Could you check a few things on this drawing? It's one solid part, dimensions in mm from its lowest x, y, z. Give positions to 0.01 mm unless a question says otherwise; leave off trailing zeros. Write each loop counter-clockwise with the first axis right and the second up, starting at its lowest first coordinate (ties: lowest second). Pieces come first, ordered by that corner, then holes. Notation, with made-up numbers: (68, -27) -> (79, -27) arc R31 ccw to (79, 7) -> close; hole circle Ø2 at (-31, -37.75). An arc over 180 degrees is marked (long way). Use CSV: the item, a comma, the result in double quotes. Start each with the question number.
(1) For pin 1 Ø1 at (x, y) = (23.5, 11.5) entering from -Z; pin 2 Ø8 at (x, z) = (10.5, 18) entering from +Y; pin 3 Ø6 at (y, z) = (9, 27) entering from -X; pin 4 Ø6 at (x, z) = (4.5, 11.5) entering from -Y, each with a flat end and sliding along its axis, tell me the tip position at first contact or that it passes through.
(2) Suppose I cut it at D-D on y = 3.5. List the corners of the cut face in (x, z) for me.
(3) Suppose I cut it at C-C on y = 26. List the corners of the cut face in (x, z) for me, plus the area to 3 significant figures.
(4) Suppose I cut it at A-A on x = 17. List the corners of the cut face in (y, z) for me, plus the area to 3 significant figures.
(5) I need wall thicknesses on L1, parallel to X at y = 14.5, z = 17; L2, parallel to Y at x = 12.5, z = 4.5; L3, parallel to Z at x = 10, y = 28. Which ranges of each line are inside material? Lowest first, please. Write a range as [from, to].
(6) If we mould it in two halves opening along Z, with no side actions, what happens to the marked faces 1, 2 and 3? For each: pulls with the +Z half, pulls with the -Z half, needs draft (parallel to the pull), parting line crosses it, or undercut.
(7) Suppose I cut it at B-B on z = 17. List the corners of the cut face in (x, y) for me, plus the area to 3 significant figures.
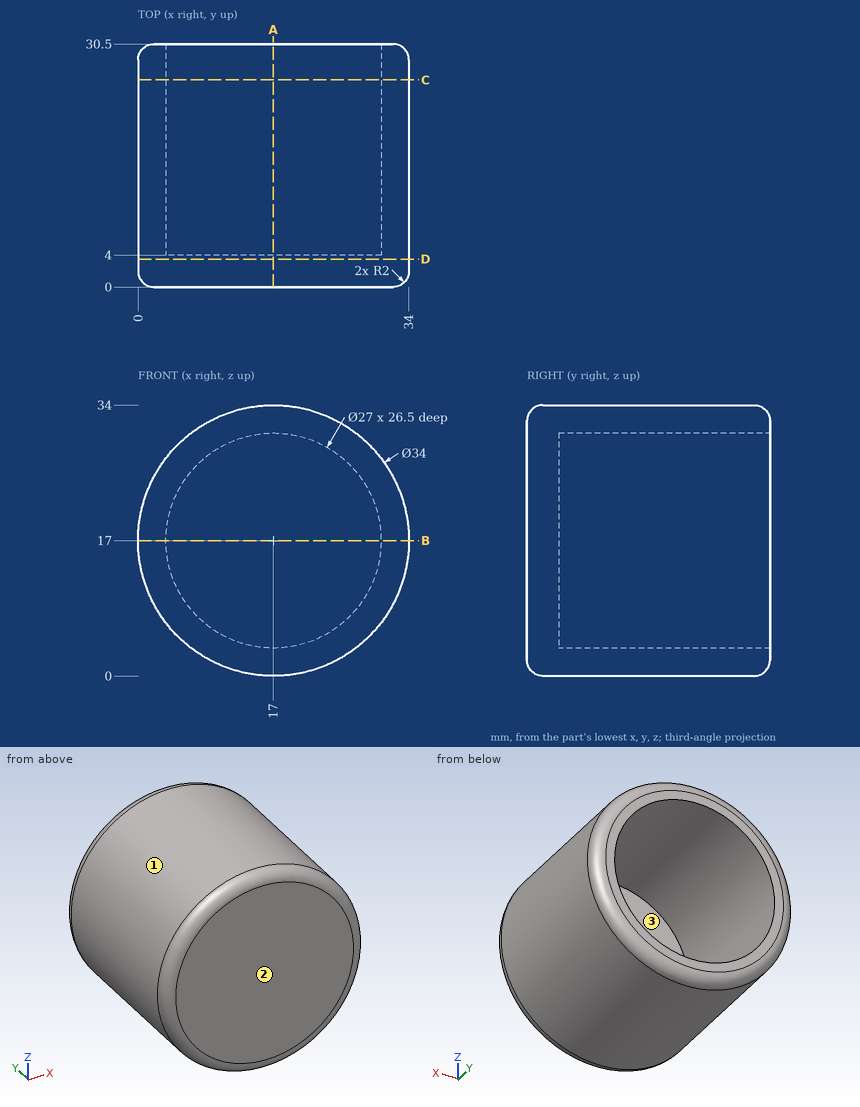
Geometry says:
1,pin 1,"z = 1.09"
1,pin 2,"y = 4"
1,pin 3,"x = 1.51"
1,pin 4,"y = 0"
2,outline,"circle Ø34 at (17, 17)"
3,outline,"circle Ø34 at (17, 17); hole circle Ø27 at (17, 17)"
3,area,"335 mm²"
4,outline,"(0, 2) arc R2 ccw to (2, 0) -> (28.5, 0) arc R2 ccw to (30.5, 2) -> (30.5, 3.5) -> (4, 3.5) -> (4, 30.5) -> (30.5, 30.5) -> (30.5, 32) arc R2 ccw to (28.5, 34) -> (2, 34) arc R2 ccw to (0, 32) -> close"
4,area,"318 mm²"
5,L1,"[0, 3.5], [30.5, 34]"
5,L2,"[0, 4]"
5,L3,"[1.51, 5.46], [28.54, 32.49]"
6,face 1,"parting line crosses it"
6,face 2,"needs draft"
6,face 3,"undercut"
7,outline,"(0, 2) arc R2 ccw to (2, 0) -> (32, 0) arc R2 ccw to (34, 2) -> (34, 28.5) arc R2 ccw to (32, 30.5) -> (30.5, 30.5) -> (30.5, 4) -> (3.5, 4) -> (3.5, 30.5) -> (2, 30.5) arc R2 ccw to (0, 28.5) -> close"
7,area,"318 mm²"
